Build history of the part. All positions in model axes, mm. A direction names the side the tool comes from. Give positions to 0.01 mm unless a question says otherwise; leave off trailing zeros. Loops run counter-clockwise (first coordinate to the right, second up) from the corner with the lowest first, then second, coordinate; pieces in that order, holes last. Notation, with made-up numbers: M 62.5,-3.5 L 100.5,-3.5 A24 ccw 100.5,9.5 Z; hole C -17.75,2.25 d2. An arc over 180 degrees is marked long. Answer in a Markdown table with one row per item. Add a question column.
```python
from build123d import *

# Parameters (mm, degrees)
SKETCH1_W           = 121.249023843
SKETCH1_H           = 101.6
SKETCH1_R           = 20.955
SKETCH1_R_2         = 3.175
BOSS_EXTRUDE1_DEPTH = 25.4
SKETCH2_R           = 6.35
CUT_EXTRUDE1_DEPTH  = 102.6
SKETCH3_W           = 31.554427073
SKETCH3_H           = 3.175
CUT_EXTRUDE2_DEPTH  = 26.4


with BuildPart() as part:
    # Sketch1 → Boss-Extrude1 (new body)
    with BuildSketch(Plane(origin=(0, 0, 0), x_dir=(1, 0, 0), z_dir=(0, 1, 0))):
        with Locations((142.575488079, 50.8)):
            Rectangle(SKETCH1_W, SKETCH1_H)
        with Locations((152.4, 50.8)):
            Circle(SKETCH1_R, mode=Mode.SUBTRACT)
        with Locations((98.1075, 50.8)):
            Circle(SKETCH1_R_2, mode=Mode.SUBTRACT)
    extrude(amount=BOSS_EXTRUDE1_DEPTH)

    # Sketch2 → Cut-Extrude1 (cut, through all)
    with BuildSketch(Plane.XY):
        with Locations((187.325, 12.7)):
            Circle(SKETCH2_R)
    extrude(amount=-CUT_EXTRUDE1_DEPTH, mode=Mode.SUBTRACT)

    # Sketch3 → Cut-Extrude2 (cut, through all)
    with BuildSketch(Plane(origin=(0, 25.4, 0), x_dir=(1, 0, 0), z_dir=(0, 1, 0))):
        with Locations((187.422786464, 50.8)):
            Rectangle(SKETCH3_W, SKETCH3_H)
    extrude(amount=-CUT_EXTRUDE2_DEPTH, mode=Mode.SUBTRACT)


solid = part.part
```
(1) Slice it at C-C, the plane x = 152.4. Give the cut face in (y, z) (3 decimals).
(2) Pull direction Z, two halves, no side cores. Call faces 1 (the flat face through (128, 0, -52)), 2 (the flat face through (142, 13, 0)), 3 (the flat face through (191, 19, -49.212)): +Z half, -Z half, draft (parallel to the pull), parting line (faces both ways), or undercut.
(3) Wall check: line 1 (Z direction, x = 180.5, y = 13); line 2 (X direction, y = 12.75, z = -50.8) (1 decimal); line 3 (Z direction, x = 152.4, y = 10.5) (3 decimals). Give the ranges that are in metal, low to high.
(4) Pin check, flat tip, straight feed: pin 1 (6 mm diameter, centred on x = 189.5, y = 9.5, fed in from +Z). Stop position of the tip, or through.
(5) Slice it at A-A, the plane y = 12.7. State how many separate pieces and enclosed holes the cut face has, then the cut area to 3 significant figures.
(6) Tool access for faces 4 (the cylindrical face through (180.98, 12.98, -24.26)), 5 (the flat face through (191, 19, -52.387)): list every direction of +Z, -Z, +X, -X, +Y, -Y with a clear straight run to the whole face (end or side of a thin tool).
(7) Slice it at B-B, the plane z = -45. Give the cut face in (x, y) (3 decimals), then the cut area to 3 significant figures.
Solution:
| question | item | result |
|---|---|---|
| 1 | outline | M 0,-101.6 L 25.4,-101.6 L 25.4,-71.755 L 0,-71.755 Z; M 0,-29.845 L 25.4,-29.845 L 25.4,0 L 0,0 Z |
| 2 | face 1 | draft |
| 2 | face 2 | +Z half |
| 2 | face 3 | undercut |
| 3 | line 1 | -101.6 to -52.39, -49.21 to 0 |
| 3 | line 2 | 82 to 94.9, 101.3 to 131.4 |
| 3 | line 3 | -101.6 to -71.755, -29.845 to 0 |
| 4 | pin 1 | z = 0 |
| 5 | separate pieces | 3 |
| 5 | enclosed holes | 1 |
| 5 | area | 9,560 mm^2 |
| 6 | face 4 | +Z, -Z |
| 6 | face 5 | +X, +Y, -Y |
| 7 | outline | M 81.951,0 L 132.264,0 L 132.264,25.4 L 81.951,25.4 Z; M 172.536,0 L 203.2,0 L 203.2,25.4 L 172.536,25.4 Z; hole C 187.325,12.7 d12.7 |
| 7 | area | 1,930 mm^2 |
